Can you work these out from the model? Positions are in its coordinate system, mm. A direction names the side the tool comes from. Round coordinates to 2 decimals unless told otherwise and drop trailing zeros. Loops run counter-clockwise (first coordinate to the right, second up) from the corner with the lowest first, then second, coordinate; pieces in that order, holes last. Notation, with made-up numbers: (-13.75, -36.75) -> (-8.75, -36.75) arc R29 ccw to (-8.75, -5.75) -> close; hole circle Ø11 at (66, 2.5). An arc over 180 degrees is marked (long way). Write item = value, one per line.
from build123d import *

# Parameters (mm, degrees)
F3_DEPTH  = 6.35
F4_DEPTH  = 3.81
F5_DEPTH  = 5.08
F7_DEPTH  = 2.54
F9_DEPTH  = 2.54
F11_DEPTH = 2.54
F13_DEPTH = 1.27
F15_R     = 1.905
F16_DEPTH = 25.4


with BuildPart() as f3:
    # F0 (on Front) → F3 (new body)
    with BuildSketch(Plane.XZ):
        Polygon((0, 0), (16.497784, 9.525), (16.497784, 28.575), (0, 38.1), (-16.497784, 28.575), (-16.497784, 9.525), align=None)
    extrude(amount=F3_DEPTH)

    # F1 (on Front) → F4 (join)
    with BuildSketch(Plane.XZ):
        Polygon((16.497784, 9.525), (0, 0), (0, -19.05), (16.497784, -28.575), (32.995568, -19.05), (32.995568, 0), align=None)
    extrude(amount=F4_DEPTH)

    # F2 (on Front) → F5 (join)
    with BuildSketch(Plane.XZ):
        Polygon((-32.995568, -19.05), (-16.497784, -28.575), (0, -19.05), (0, 0), (-16.497784, 9.525), (-32.995568, 0), align=None)
    extrude(amount=F5_DEPTH)

    # F6 (on face) → F7 (cut)
    with BuildSketch(Plane.XZ.offset(6.35)):
        Polygon((-10.147784, 24.908826), (-10.147784, 13.191174), (0, 7.332348), (10.147784, 13.191174), (10.147784, 24.908826), (0, 30.767652), align=None)
    extrude(amount=-F7_DEPTH, mode=Mode.SUBTRACT)

    # F8 (on face) → F9 (cut)
    with BuildSketch(Plane.XZ.offset(5.08)):
        Polygon((-16.497784, 2.192652), (-26.645568, -3.666174), (-26.645568, -15.383826), (-16.497784, -21.242652), (-6.35, -15.383826), (-6.35, -3.666174), align=None)
    extrude(amount=-F9_DEPTH, mode=Mode.SUBTRACT)

    # F10 (on face) → F11 (cut)
    with BuildSketch(Plane.XZ.offset(3.81)):
        Polygon((16.497784, 2.192652), (6.35, -3.666174), (6.35, -15.383826), (16.497784, -21.242652), (26.645568, -15.383826), (26.645568, -3.666174), align=None)
    extrude(amount=-F11_DEPTH, mode=Mode.SUBTRACT)

    # F15 (on face) → F16 (cut)
    with BuildSketch(Plane.XZ.offset(6.35)):
        with Locations((0, 33.614568)):
            Circle(F15_R)
    extrude(amount=-F16_DEPTH, mode=Mode.SUBTRACT)


with BuildPart() as f13:
    # F12 (on Front) → F13 (new body)
    with BuildSketch(Plane.XZ):
        Polygon((0, -19.372597), (-7.288163, -23.370054), (0, -30.658217), (7.288163, -23.370054), align=None)
    extrude(amount=F13_DEPTH)


solid = f3.part
1. I need wall thicknesses on line 1 (X direction, y = -3.5, z = -8.5); line 2 (X direction, y = -3.75, z = -3); line 3 (Z direction, x = 0, y = -1.25). Which ranges of each line are inside material? Lowest first, please. Write a range as [from, to].
Entries:
line_1 = [-33, -26.65], [-6.35, 6.35], [26.65, 33]
line_2 = [-33, -25.49], [-7.5, 7.5], [25.49, 33]
line_3 = [-19.05, 31.71], [35.52, 38.1]
2. We'd pull the mould along Z, two halves only. Please class faces 4 (the flat face through (-16.498, -3, 19)), 5 (the flat face through (-24.63, -2.5, 4.83)), 6 (the flat face through (8.133, -1.878, -23.746)), 7 (the flat face through (5, -5.1, 10.22)): released by +Z, released by -Z, zero draft, split by the parting line, or undercut.
Entries:
face_4 = zero draft
face_5 = released by +Z
face_6 = released by -Z
face_7 = undercut
3. I'm going to push flat-ended pins straight in: pin 1 (3 mm diameter, centred on y = -5, z = 16.5, fed in from +X); pin 2 (1.4 mm diameter, centred on y = -4, z = -12.5, fed in from +X); pin 3 (22.5 mm diameter, centred on x = 20.5, z = -11.5, fed in from -Y); pin 4 (3 mm diameter, centred on y = -2, z = 23, fed in from -X). Where does each tip first touch, or does it pass through?
Entries:
pin_1 = 16.5
pin_2 = 33
pin_3 = -3.81
pin_4 = -16.5
4. Suppose I cut it at A-A, the plane z = -14. List the corners of the cut face in (x, y) for me.
Entries:
outline = (-33, -5.08) -> (-26.65, -5.08) -> (-26.65, -2.54) -> (-6.35, -2.54) -> (-6.35, -5.08) -> (0, -5.08) -> (0, -3.81) -> (6.35, -3.81) -> (6.35, -1.27) -> (26.65, -1.27) -> (26.65, -3.81) -> (33, -3.81) -> (33, 0) -> (-33, 0) -> close
5. Suppose I cut it at B-B, the plane x = 18. List the corners of the cut face in (y, z) for me, and give its area (3 significant figures).
Entries:
outline = (-3.81, -27.71) -> (0, -27.71) -> (0, 8.66) -> (-3.81, 8.66) -> (-3.81, 1.33) -> (-1.27, 1.33) -> (-1.27, -20.38) -> (-3.81, -20.38) -> close
area = 83.4 mm²
6. Suppose I cut it at D-D, the plane x = 8. List the corners of the cut face in (y, z) for me.
Entries:
outline = (-6.35, 4.62) -> (-3.81, 4.62) -> (-3.81, -2.71) -> (-1.27, -2.71) -> (-1.27, -16.34) -> (-3.81, -16.34) -> (-3.81, -23.67) -> (0, -23.67) -> (0, 33.48) -> (-6.35, 33.48) -> (-6.35, 26.15) -> (-3.81, 26.15) -> (-3.81, 11.95) -> (-6.35, 11.95) -> close
7. For faces 1 (the flat face through (26.646, -3, -10)), 2 (the flat face through (16.498, -3, 19)), 3 (the cylindrical face through (-0.413, -3.219, 31.755)), which set-ups out of +Z, -Z, +X, -X, +Y, -Y let a thin tool reach every point of the face, with its end or its side?
Entries:
face_1 = -Y
face_2 = +Z, +X, +Y, -Y
face_3 = +Y, -Y
8. Suppose I cut it at C-C, the plane x = -24.5. List the corners of the cut face in (y, z) for me.
Entries:
outline = (-5.08, -23.95) -> (0, -23.95) -> (0, 4.9) -> (-5.08, 4.9) -> (-5.08, -2.43) -> (-2.54, -2.43) -> (-2.54, -16.62) -> (-5.08, -16.62) -> close
